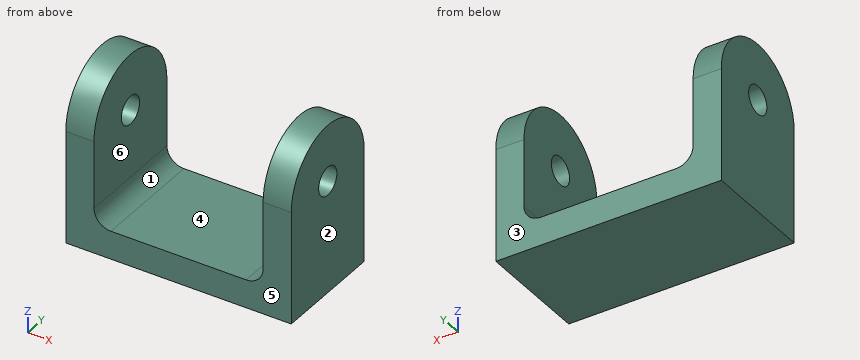
Solid Edge part; units mm, degrees
sketch "Sketch1" plane through (0, 0, 0) normal (0, -1, 0) x (1, 0, 0)
  line L0 (15, 30) -> (15, 5)
  line L1 (15, 5) -> (0, 5)
  line L2 (-15, 5) -> (0, 5)
  line L3 (-15, 30) -> (-15, 5)
  line L4 (-20, 30) -> (-15, 30)
  line L5 (-20, 0) -> (-20, 30)
  line L6 (0, 0) -> (-20, 0)
  line L7 (0, 0) -> (20, 0)
  line L8 (20, 0) -> (20, 30)
  line L9 (20, 30) -> (15, 30)
extrude "ProtrusiónExtruida_1" add sketch "Sketch1" along normal mid plane 20
sketch "Sketch2" plane through (20, 0, 15) normal (1, 0, 0) x (0, 1, 0)
  line L0 (0, 15) -> (10, 15)
  line L1 (10, 5) -> (10, 15)
  arc A0 (0, 15) -> (10, 5) centre (0, 5) cw
  line L2 (-10, 5) -> (-10, 15)
  line L3 (-10, 15) -> (0, 15)
  arc A1 (-10, 5) -> (0, 15) centre (0, 5) cw
  circle A2 centre (0, 5) radius 2.5
extrude "VaciadoExtruido_1" cut sketch "Sketch2" along normal mid plane 152.2925
fillet "Redondeo_1" radius 3 2 edges at (-15, 0, 5) (15, 0, 5)
properties material "PLA"
The model under review builds one solid part; all positions refer to its coordinate system, in mm. Face numbers are marked on the shaded views. A direction names the side the tool comes from. Give positions to 0.01 mm unless a question says otherwise; leave off trailing zeros. Order: outer loops, then holes, each group sorted by start corner. A loop starts at its lowest first (then second) coordinate and runs counter-clockwise, first axis right, second up. Notation, with made-up numbers: M 71.5,-12.75 L 122.5,-12.75 A29 ccw 122.5,23.25 Z; hole C -38.5,30 d1. An arc over 180 degrees is marked long. Answer in a Markdown table with one row per item. Add a question column.
1. Mouldability with a two-part tool opening along X and no side actions: class the marked faces 1, 2, 3 and 4 as released by +X, released by -X, zero draft, split by the parting line, or undercut.
2. Add section C-C on x = -8. State the section outline as (y, z) points, plus the area to 3 significant figures.
3. Add section D-D on y = 4.5. State the section outline as (x, z) points, plus the area to 3 significant figures.
4. Add section B-B on z = 14. State the section outline as (x, y) points.
5. Add section A-A on y = 0. State the section outline as (x, z) points.
6. Machinability: for the marked faces 5 and 6, which of the approach directions +Z, -Z, +X, -X, +Y, -Y give a long, thin tool a straight path to every point of the face, cutting with its end or side? Answer none if there is none.
7. To check wall thickness, follow line 1 along X through (y, z) = (-5, 24.5); line 2 along Z through (x, y) = (18.25, 0); line 3 along Z through (x, y) = (8, 6.5). State the ranges of each line that lie inside material, in increasing order.
8. For pin 1 Ø5 at (x, y) = (-15.5, 6) entering from +Z; pin 2 Ø10 at (x, y) = (2.5, -2) entering from +Z; pin 3 Ø8 at (x, y) = (-10.5, -7) entering from +Z, all flat-tipped, find the tip position at first contact; note any pin that passes through.
The answers:
| question | item | result |
|---|---|---|
| 1 | face 1 | undercut |
| 1 | face 2 | released by +X |
| 1 | face 3 | zero draft |
| 1 | face 4 | undercut |
| 2 | outline | M -10,0 L 10,0 L 10,5 L -10,5 Z |
| 2 | area | 100 mm2 |
| 3 | outline | M -20,0 L 20,0 L 20,28.93 L 15,28.93 L 15,8 A3 cw 12,5 L -12,5 A3 cw -15,8 L -15,28.93 L -20,28.93 Z |
| 3 | area | 443 mm2 |
| 4 | outline | M -20,-10 L -15,-10 L -15,10 L -20,10 Z; M 15,-10 L 20,-10 L 20,10 L 15,10 Z |
| 5 | outline | M -20,0 L 20,0 L 20,17.5 L 15,17.5 L 15,8 A3 cw 12,5 L -12,5 A3 cw -15,8 L -15,17.5 L -20,17.5 Z; M -20,22.5 L -15,22.5 L -15,30 L -20,30 Z; M 15,22.5 L 20,22.5 L 20,30 L 15,30 Z |
| 6 | face 5 | +Z, -Z, +X, -X, -Y |
| 6 | face 6 | +Z, +Y, -Y |
| 7 | line 1 | -20 to -15, 15 to 20 |
| 7 | line 2 | 0 to 17.5, 22.5 to 30 |
| 7 | line 3 | 0 to 5 |
| 8 | pin 1 | z = 29.37 |
| 8 | pin 2 | z = 5 |
| 8 | pin 3 | z = 6.34 |
